Could you check a few things on this drawing? It's one solid part, dimensions in mm from its lowest x, y, z. A direction names the side the tool comes from. Give positions to 0.01 mm unless a question says otherwise; leave off trailing zeros. Loops run counter-clockwise (first coordinate to the right, second up) from the corner with the lowest first, then second, coordinate; pieces in that order, holes last. Notation, with made-up numbers: M 61.5,84 L 110.5,84 A23 ccw 110.5,123 Z; hole C -28,82.5 d11. An arc over 180 degrees is marked long. Answer in a Markdown table with one row per item. Add a question column.
1. If we section it at A-A on z = 7.5: List the corners of the cut face in (x, y) for me, then the cut area to 3 significant figures.
2. If we section it at C-C on y = 29: List the corners of the cut face in (x, z) for me, then the cut area to 3 significant figures.
3. If we section it at B-B on x = 8.5: List the corners of the cut face in (y, z) for me.
4. Which directions (+Z, -Z, +X, -X, +Y, -Y) give clear straight access to the entire face, cutting with the end or side of a thin tool? Please do the marked faces 1, 2 and 3.
5. If we section it at D-D on x = 14.25: List the corners of the cut face in (y, z) for me.
6. I'm going to push flat-ended pins straight in: pin 1 Ø6 at (y, z) = (102, 21.5) entering from -X; pin 2 Ø12.5 at (y, z) = (93.5, 17) entering from +X; pin 3 Ø12.5 at (y, z) = (8.5, 8.5) entering from -X; pin 4 Ø5 at (x, z) = (19.5, 14) entering from +Y. Where does each tip first touch, or does it pass through?
7. I need wall thicknesses on line 1 along Y through (x, z) = (7, 12.5) (1 decimal); line 2 along X through (y, z) = (68, 6.5); line 3 along X through (y, z) = (27.5, 7.75). Which ranges of each line are inside material? Lowest first, please. Write a range as from..to.
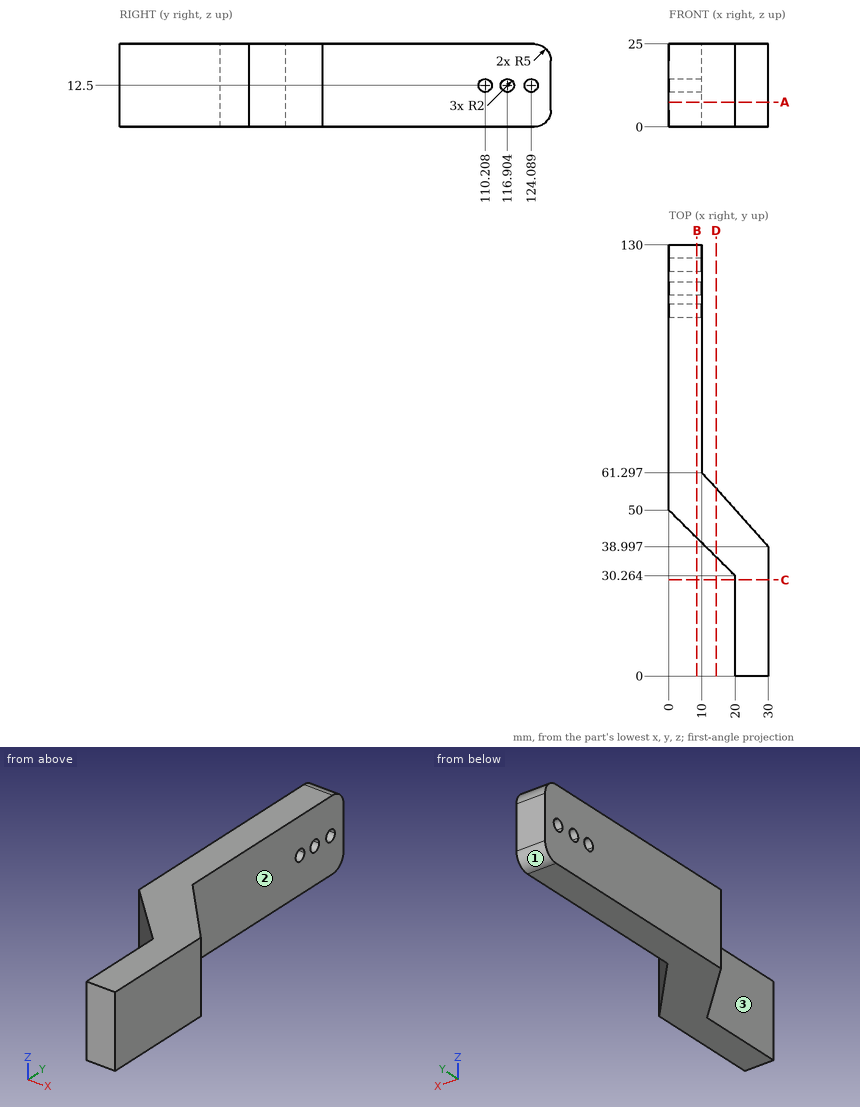
Results:
| question | item | result |
|---|---|---|
| 1 | outline | M 0,50 L 20,30.26 L 20,0 L 30,0 L 30,39 L 10,61.3 L 10,130 L 0,130 Z |
| 1 | area | 1,500 mm2 |
| 2 | outline | M 20,0 L 30,0 L 30,25 L 20,25 Z |
| 2 | area | 250 mm2 |
| 3 | outline | M 41.61,0 L 125,0 A5 ccw 130,5 L 130,20 A5 ccw 125,25 L 41.61,25 Z; hole C 110.21,12.5 d4; hole C 116.9,12.5 d4; hole C 124.09,12.5 d4 |
| 4 | face 1 | -Z, +X, -X, +Y |
| 4 | face 2 | +Z, -Z, +X, +Y |
| 4 | face 3 | +Z, -Z, -X, -Y |
| 5 | outline | M 35.94,0 L 56.56,0 L 56.56,25 L 35.94,25 Z |
| 6 | pin 1 | x = 0 |
| 6 | pin 2 | x = 10 |
| 6 | pin 3 | x = 20 |
| 6 | pin 4 | y = 53.49 |
| 7 | line 1 | 43.1..108.2, 112.2..114.9, 118.9..122.1, 126.1..130 |
| 7 | line 2 | 0..10 |
| 7 | line 3 | 20..30 |
